Autodesk Fusion 360 part; units mm, degrees
sketch "Sketch1" plane through (0, 0, 0) normal (1, 0, 0) x (0, 1, 0)
  line L0 (0, 0) -> (28, 0)
  line L1 (28, 0) -> (28, 28)
  line L2 (28, 28) -> (22, 28)
  line L3 (22, 28) -> (22, 24)
  line L4 (0, 0) -> (0, 6)
  line L5 (0, 6) -> (4, 6)
  line L6 (4, 6) -> (22, 24)
  dimension "d1" = 28
  dimension "d2" = 28
extrude "Extrude1" add sketch "Sketch1" along normal blind 3
sketch "Sketch2" plane through (3, 0, 0) normal (1, 0, 0) x (0, 1, 0)
  line L0 (0, 0) -> (28, 0)
  line L1 (28, 0) -> (28, 28)
  line L2 (28, 28) -> (22, 28)
  line L3 (22, 28) -> (22, 24)
  line L4 (22, 24) -> (4, 6)
  line L5 (4, 6) -> (0, 6)
  line L6 (0, 6) -> (0, 0)
  line L7 (0, 0) -> (28, 0)
  line L8 (28, 0) -> (28, 4)
  line L9 (24, 4) -> (0, 4)
  line L10 (0, 4) -> (0, 0)
  line L11 (28, 28) -> (24, 28)
  line L12 (24, 28) -> (24, 4)
  line L13 (24, 0) -> (28, 0)
  line L14 (28, 0) -> (28, 28)
  dimension "d5" = 4
  dimension "d6" = 28
extrude "Extrude2" add sketch "Sketch2" along normal blind 14 contours L0 L1 L2 L6 L7 L8 L9 L10 L11 L12 L13 L14
sketch "Sketch3" plane through (17, 0, 0) normal (1, 0, 0) x (0, 1, 0)
  line L0 (28, 0) -> (28, 28)
  line L1 (28, 28) -> (24, 28)
  line L2 (24, 28) -> (24, 4)
  line L3 (24, 4) -> (0, 4)
  line L4 (0, 4) -> (0, 0)
  line L5 (0, 0) -> (28, 0)
  line L6 (0, 0) -> (28, 0)
  line L7 (28, 28) -> (28, 0)
  line L8 (28, 28) -> (22, 28)
  line L9 (22, 28) -> (22, 24)
  line L10 (22, 24) -> (4, 6)
  line L11 (4, 6) -> (0, 6)
  line L12 (0, 6) -> (0, 0)
sketch "Sketch4" plane through (17, 0, 0) normal (1, 0, 0) x (0, 1, 0)
extrude "Extrude3" add sketch "Sketch3" along normal blind 3
sketch "Sketch5" plane through (0, 24, 0) normal (0, -1, 0) x (1, 0, 0)
  line L0 (3, 28) -> (3, 4)
  line L1 (3, 4) -> (17, 4)
  line L2 (17, 4) -> (17, 28)
  line L3 (17, 28) -> (3, 28)
fillet "Fillet1" radius 1 1 edges at (1.5, 22, 28)
fillet "Fillet2" radius 1 1 edges at (18.5, 22, 28)
fillet "Fillet3" radius 1 1 edges at (1.5, 0, 6)
fillet "Fillet4" radius 1 1 edges at (18.5, 0, 6)
fillet "Fillet5" radius 1 1 edges at (1.5, 4, 6)
fillet "Fillet6" radius 1 1 edges at (18.5, 4, 6)
fillet "Fillet7" radius 1 1 edges at (1.5, 22, 24)
fillet "Fillet8" radius 1 1 edges at (18.5, 22, 24)
sketch "Sketch6" plane through (0, 24, 0) normal (0, -1, 0) x (1, 0, 0)
  line L0 (11, 19) -> (9, 19)
  line L1 (7, 17) -> (7, 11)
  line L2 (9, 9) -> (11, 9)
  line L3 (13, 11) -> (13, 17)
  line L4 (13, 19) -> (7, 9) construction
  line L5 (7, 19) -> (13, 9) construction
  arc A0 (9, 19) -> (7, 17) centre (9, 17) ccw
  arc A1 (13, 17) -> (11, 19) centre (11, 17) ccw
  arc A2 (11, 9) -> (13, 11) centre (11, 11) ccw
  arc A3 (7, 11) -> (9, 9) centre (9, 11) ccw
  point P0 (10, 14)
  dimension "d27" = 6
  dimension "d28" = 10
  dimension "d29" = 2
extrude "Extrude4" cut sketch "Sketch6" against normal blind 7
sketch "Sketch7" plane through (0, 0, 4) normal (0, 0, 1) x (-1, 0, 0)
  line L0 (-3, -24) -> (-3, 0)
  line L1 (-3, 0) -> (-17, 0)
  line L2 (-17, 0) -> (-17, -24)
  line L3 (-17, -24) -> (-3, -24)
  line L4 (-9, -9) -> (-11, -9)
  line L5 (-13, -11) -> (-13, -17)
  line L6 (-11, -19) -> (-9, -19)
  line L7 (-7, -17) -> (-7, -11)
  line L8 (-7, -9) -> (-13, -19) construction
  line L9 (-13, -9) -> (-7, -19) construction
  arc A0 (-9, -19) -> (-7, -17) centre (-9, -17) ccw
  arc A1 (-7, -11) -> (-9, -9) centre (-9, -11) ccw
  arc A2 (-13, -17) -> (-11, -19) centre (-11, -17) ccw
  arc A3 (-11, -9) -> (-13, -11) centre (-11, -11) ccw
  point P0 (-10, -14)
  dimension "d32" = 6
  dimension "d33" = 10
  dimension "d34" = 2
extrude "Extrude5" cut sketch "Sketch7" against normal blind 4 contours L4 L5 L6 L7 A0 A1 A2 A3
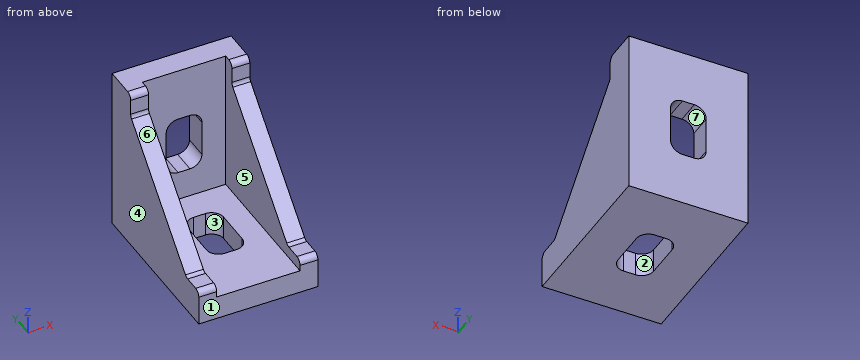
Read the model definition and answer for the solid it produces. Units are mm, in the model's axes. Face numbers are marked on the shaded views. A direction names the side the tool comes from. Coordinates: 2 decimals unless noted, no trailing zeros. Loops run counter-clockwise (first coordinate to the right, second up) from the corner with the lowest first, then second, coordinate; pieces in that order, holes last.
Q1. The part is cut by section C-C on x = 9.5. Write down the section's boundary in (y, z).
Q2. Consider probe 1 along X at (y, z) = (16, 2); probe 2 along X at (y, z) = (12, 8.75); probe 3 along Y at (x, z) = (7.25, 21.25). Determine where each line is inside the solid, lowest interval first.
Q3. Each of these flat-tipped pins is pushed along its axis until it touches: pin 1 Ø3 at (x, z) = (7.5, 24.5) entering from -Y; pin 2 Ø10 at (x, z) = (16, 16) entering from -Y; pin 3 Ø3 at (x, z) = (2, 26) entering from -Y. Where does it stop, or does it pass through?
Q4. The part is cut by section D-D on y = 5.75. Write down the section's boundary in (x, z).
Q5. The part is cut by section A-A on y = 15.25. Write down the section's boundary in (x, z).
Q6. The mould has two halves that part along X. Classify the marked faces 1, 2, 3 and 4: +X half, -X half, draft (parallel to the pull), parting line (faces both ways), or undercut.
Q7. Which of the six approach directions +Z, -Z, +X, -X, +Y, -Y give full straight-line access (tool end or side, diameter ignored) to the marked faces 5, 6 and 7?
Q8. The part is cut by section B-B on z = 16. Write down the section's boundary in (x, y).
Results below:
1. outline: (0, 0) - (9, 0) - (9, 4) - (0, 4) - close; (19, 0) - (28, 0) - (28, 9) - (24, 9) - (24, 4) - (19, 4) - close; (24, 19) - (28, 19) - (28, 28) - (24, 28) - close
2. probe 1: x = 0 to 7, 13 to 20
2. probe 2: x = 0 to 3, 17 to 20
2. probe 3: y = 24 to 28
3. pin 1: stops at y = 24
3. pin 2: stops at y = 9.1
3. pin 3: stops at y = 22
4. outline: (0, 0) - (20, 0) - (20, 7.75) - (17, 7.75) - (17, 4) - (3, 4) - (3, 7.75) - (0, 7.75) - close
5. outline: (0, 0) - (7, 0) - (7, 4) - (3, 4) - (3, 17.25) - (0, 17.25) - close; (13, 0) - (20, 0) - (20, 17.25) - (17, 17.25) - (17, 4) - (13, 4) - close
6. face 1: draft
6. face 2: undercut
6. face 3: undercut
6. face 4: -X half
7. face 5: +Z, -Y
7. face 6: +Z, +X, -X, -Y
7. face 7: +Y, -Y
8. outline: (0, 14) - (3, 14) - (3, 24) - (7, 24) - (7, 28) - (0, 28) - close; (13, 24) - (17, 24) - (17, 14) - (20, 14) - (20, 28) - (13, 28) - close
